from build123d import *

# Parameters (mm, degrees)
SKETCH_1_R          = 10
EXTRUDE_1_DEPTH     = 30
SKETCH_2_R          = 1.85
CUT_EXTRUDE_1_DEPTH = 34.166247904
SKETCH_3_R          = 1.85
SKETCH_3_R_2        = 1.6
EXTRUDE_2_DEPTH     = 15
CUT_EXTRUDE_START   = -15
SKETCH_4_R          = 2.5
SKETCH_4_R_2        = 1.85
CUT_EXTRUDE_2_DEPTH = 15
EXTRUDE_START       = -15
SKETCH_5_R          = 1.85
SKETCH_5_R_2        = 1.6
EXTRUDE_3_DEPTH     = 15
SKETCH_6_R          = 2.5
CUT_EXTRUDE_4_DEPTH = 15
SKETCH_8_W          = 25
SKETCH_8_H          = 25
SKETCH_8_R          = 10
EXTRUDE_4_DEPTH     = 3
FILLET_1_R          = 4
FILLET_6_R          = 12.5
FILLET_7_R          = 12.5
FILLET_8_R          = 12.5
FILLET_9_R          = 12.5
EXTRUDE_START_2     = -25
SKETCH_9_R          = 2.5
EXTRUDE_6_DEPTH     = 25
SKETCH_10_R         = 1.9
CUT_EXTRUDE_5_DEPTH = 10
SKETCH_11_R         = 3
CUT_EXTRUDE_6_DEPTH = 15
EXTRUDE_START_3     = 20
SKETCH_13_R         = 10
SKETCH_13_R_2       = 3
SKETCH_13_R_3       = 1.9
EXTRUDE_7_DEPTH     = 20


# Some blends are built 0.0001 mm under size
with BuildPart() as part:
    # 草图1 → 凸台-拉伸1 (new body)
    with BuildSketch(Plane(origin=(0, 0, 0), x_dir=(1, 0, 0), z_dir=(0, 1, 0))):
        with Locations(Location((0, 0, 0), (0, 0, 270))):
            Circle(SKETCH_1_R)
    extrude(amount=EXTRUDE_1_DEPTH)

    # 草图2 → 切除-拉伸1 (cut, through all)
    with BuildSketch(Plane(origin=(0, 30, 0), x_dir=(1, 0, 0), z_dir=(0, 1, 0))):
        with Locations(Location((0, 6, 0), (0, 0, 270))):
            Circle(SKETCH_2_R)
        with Locations(Location((5.196152423, 3, 0), (0, 0, 270))):
            Circle(SKETCH_2_R)
        with Locations(Location((5.196152423, -3, 0), (0, 0, 270))):
            Circle(SKETCH_2_R)
        with Locations(Location((0, -6, 0), (0, 0, 270))):
            Circle(SKETCH_2_R)
        with Locations(Location((-5.196152423, -3, 0), (0, 0, 270))):
            Circle(SKETCH_2_R)
        with Locations(Location((-5.196152423, 3, 0), (0, 0, 270))):
            Circle(SKETCH_2_R)
    extrude(amount=-CUT_EXTRUDE_1_DEPTH, mode=Mode.SUBTRACT)

    # 草图3 → 凸台-拉伸2 (add)
    # profile 1 of 3: a face of its own
    with BuildSketch(Plane(origin=(0, 30, 0), x_dir=(1, 0, 0), z_dir=(0, 1, 0))):
        with Locations(Location((0, 6, 0), (0, 0, 270))):
            Circle(SKETCH_3_R)
        with Locations(Location((0, 6, 0), (0, 0, 270))):
            Circle(SKETCH_3_R_2, mode=Mode.SUBTRACT)
    # profile 2 of 3: a face of its own
    with BuildSketch(Plane(origin=(0, 30, 0), x_dir=(1, 0, 0), z_dir=(0, 1, 0))):
        with Locations(Location((-5.196152423, -3, 0), (0, 0, 270))):
            Circle(SKETCH_3_R)
        with Locations(Location((-5.196152423, -3, 0), (0, 0, 270))):
            Circle(SKETCH_3_R_2, mode=Mode.SUBTRACT)
    # profile 3 of 3: a face of its own
    with BuildSketch(Plane(origin=(0, 30, 0), x_dir=(1, 0, 0), z_dir=(0, 1, 0))):
        with Locations(Location((5.196152423, -3, 0), (0, 0, 270))):
            Circle(SKETCH_3_R)
        with Locations(Location((5.196152423, -3, 0), (0, 0, 270))):
            Circle(SKETCH_3_R_2, mode=Mode.SUBTRACT)
    extrude(amount=-EXTRUDE_2_DEPTH)

    # 草图4 → 切除-拉伸2 (cut)
    # profile 1 of 3: a face of its own
    with BuildSketch(Plane.XZ.offset(CUT_EXTRUDE_START)):
        with Locations(Location((-5.196152423, 3, 0), (0, 0, 270))):
            Circle(SKETCH_4_R)
        with Locations((-5.196152423, 3)):
            Circle(SKETCH_4_R_2, mode=Mode.SUBTRACT)
    # profile 2 of 3: a face of its own
    with BuildSketch(Plane.XZ.offset(CUT_EXTRUDE_START)):
        with Locations(Location((5.196152423, 3, 0), (0, 0, 270))):
            Circle(SKETCH_4_R)
        with Locations((5.196152423, 3)):
            Circle(SKETCH_4_R_2, mode=Mode.SUBTRACT)
    # profile 3 of 3: a face of its own
    with BuildSketch(Plane.XZ.offset(CUT_EXTRUDE_START)):
        with Locations(Location((0, -6, 0), (0, 0, 270))):
            Circle(SKETCH_4_R)
        with Locations((0, -6)):
            Circle(SKETCH_4_R_2, mode=Mode.SUBTRACT)
    extrude(amount=CUT_EXTRUDE_2_DEPTH, mode=Mode.SUBTRACT)

    # 草图5 → 凸台-拉伸3 (add)
    # profile 1 of 3: a face of its own
    with BuildSketch(Plane.XZ.offset(EXTRUDE_START)):
        with Locations(Location((0, 6, 0), (0, 0, 90))):
            Circle(SKETCH_5_R)
        with Locations(Location((0, 6, 0), (0, 0, 270))):
            Circle(SKETCH_5_R_2, mode=Mode.SUBTRACT)
    # profile 2 of 3: a face of its own
    with BuildSketch(Plane.XZ.offset(EXTRUDE_START)):
        with Locations(Location((-5.196152423, -3, 0), (0, 0, 90))):
            Circle(SKETCH_5_R)
        with Locations(Location((-5.196152423, -3, 0), (0, 0, 270))):
            Circle(SKETCH_5_R_2, mode=Mode.SUBTRACT)
    # profile 3 of 3: a face of its own
    with BuildSketch(Plane.XZ.offset(EXTRUDE_START)):
        with Locations(Location((5.196152423, -3, 0), (0, 0, 90))):
            Circle(SKETCH_5_R)
        with Locations(Location((5.196152423, -3, 0), (0, 0, 270))):
            Circle(SKETCH_5_R_2, mode=Mode.SUBTRACT)
    extrude(amount=EXTRUDE_3_DEPTH)

    # 草图6 → 切除-拉伸4 (cut)
    with BuildSketch(Plane(origin=(0, 30, 0), x_dir=(1, 0, 0), z_dir=(0, 1, 0))):
        with Locations(Location((-5.196152423, 3, 0), (0, 0, 270))):
            Circle(SKETCH_6_R)
        with Locations(Location((5.196152423, 3, 0), (0, 0, 270))):
            Circle(SKETCH_6_R)
        with Locations(Location((0, -6, 0), (0, 0, 270))):
            Circle(SKETCH_6_R)
    extrude(amount=-CUT_EXTRUDE_4_DEPTH, mode=Mode.SUBTRACT)

    # 草图8 → 凸台-拉伸4 (add)
    with BuildSketch(Plane.XZ):
        Rectangle(SKETCH_8_W, SKETCH_8_H)
        with Locations(Location((0, 0, 0), (0, 0, 270))):
            Circle(SKETCH_8_R, mode=Mode.SUBTRACT)
    extrude(amount=-EXTRUDE_4_DEPTH)

    # 圆角1
    # the kernel refuses this fillet: 4 mm, written as the material it adds along each edge
    with BuildSketch(Plane(origin=(0, 3, 0), x_dir=(0, 0, 1), z_dir=(-1, 0, 0))) as fillet_1_piece_1_section:
        with BuildLine():
            CenterArc((10 + FILLET_1_R, FILLET_1_R), FILLET_1_R, 180, 90)
            Line((10 + FILLET_1_R, 0), (10, 0))
            Line((10, 0), (10, FILLET_1_R))
        make_face()
    fillet_1_piece_1 = revolve(axis=Axis((0, 3, 0), (0, 1, 0)), mode=Mode.PRIVATE)
    fillet_1_piece_1 = split(fillet_1_piece_1, bisect_by=Plane(origin=(-12.5, 4.125745955, -11.125745955), z_dir=(1, 0, 0)), keep=Keep.TOP, mode=Mode.PRIVATE)
    fillet_1_piece_1 = split(fillet_1_piece_1, bisect_by=Plane(origin=(0, 4.125745955, 12.5), z_dir=(0, 0, -1)), keep=Keep.TOP, mode=Mode.PRIVATE)
    fillet_1_piece_1 = split(fillet_1_piece_1, bisect_by=Plane(origin=(12.5, 4.125745955, -11.125745955), z_dir=(-1, 0, 0)), keep=Keep.TOP, mode=Mode.PRIVATE)
    fillet_1_piece_1 = split(fillet_1_piece_1, bisect_by=Plane(origin=(0, 4.125745955, -12.5), z_dir=(0, 0, 1)), keep=Keep.TOP, mode=Mode.PRIVATE)
    add(fillet_1_piece_1)

    # 圆角6
    fillet_6_edges = [part.edges().sort_by_distance(p)[0] for p in [
        (12.5, 1.5, 12.5),
    ]]
    fillet(fillet_6_edges, radius=FILLET_6_R)

    # 圆角7
    fillet_7_edges = [part.edges().sort_by_distance(p)[0] for p in [
        (-12.5, 1.5, 12.5),
    ]]
    fillet(fillet_7_edges, radius=FILLET_7_R - 0.0001)  # a hair under: the kernel refuses the full size

    # 圆角8
    fillet_8_edges = [part.edges().sort_by_distance(p)[0] for p in [
        (-12.5, 1.5, -12.5),
    ]]
    fillet(fillet_8_edges, radius=FILLET_8_R)

    # 圆角9
    fillet_9_edges = [part.edges().sort_by_distance(p)[0] for p in [
        (12.5, 1.5, -12.5),
    ]]
    fillet(fillet_9_edges, radius=FILLET_9_R - 0.0001)  # a hair under: the kernel refuses the full size

    # 草图9 → 凸台-拉伸6 (add)
    with BuildSketch(Plane.XZ.offset(EXTRUDE_START_2)):
        with Locations((5.196152423, 3)):
            Circle(SKETCH_9_R)
        with Locations((-5.196152423, 3)):
            Circle(SKETCH_9_R)
        with Locations((0, -6)):
            Circle(SKETCH_9_R)
    extrude(amount=EXTRUDE_6_DEPTH)

    # 草图10 → 切除-拉伸5 (cut)
    with BuildSketch(Plane(origin=(0, 30, 0), x_dir=(1, 0, 0), z_dir=(0, 1, 0))):
        with Locations(Location((0, 6, 0), (0, 0, 270))):
            Circle(SKETCH_10_R)
        with Locations(Location((-5.196152423, -3, 0), (0, 0, 270))):
            Circle(SKETCH_10_R)
        with Locations(Location((5.196152423, -3, 0), (0, 0, 270))):
            Circle(SKETCH_10_R)
    extrude(amount=-CUT_EXTRUDE_5_DEPTH, mode=Mode.SUBTRACT)

    # 草图11 → 切除-拉伸6 (cut)
    with BuildSketch(Plane(origin=(0, 30, 0), x_dir=(1, 0, 0), z_dir=(0, 1, 0))):
        with Locations(Location((-5.196152423, 3, 0), (0, 0, 270))):
            Circle(SKETCH_11_R)
        with Locations(Location((5.196152423, 3, 0), (0, 0, 270))):
            Circle(SKETCH_11_R)
        with Locations(Location((0, -6, 0), (0, 0, 270))):
            Circle(SKETCH_11_R)
    extrude(amount=-CUT_EXTRUDE_6_DEPTH, mode=Mode.SUBTRACT)

    # 草图13 → 凸台-拉伸7 (add)
    with BuildSketch(Plane(origin=(0, 30, 0), x_dir=(1, 0, 0), z_dir=(0, 1, 0)).offset(EXTRUDE_START_3)):
        with Locations(Location((0, 0, 0), (0, 0, 270))):
            Circle(SKETCH_13_R)
        with Locations(Location((-5.196152423, 3, 0), (0, 0, 270))):
            Circle(SKETCH_13_R_2, mode=Mode.SUBTRACT)
        with Locations(Location((0, 6, 0), (0, 0, 270))):
            Circle(SKETCH_13_R_3, mode=Mode.SUBTRACT)
        with Locations(Location((5.196152423, 3, 0), (0, 0, 270))):
            Circle(SKETCH_13_R_2, mode=Mode.SUBTRACT)
        with Locations(Location((0, -6, 0), (0, 0, 270))):
            Circle(SKETCH_13_R_2, mode=Mode.SUBTRACT)
        with Locations(Location((5.196152423, -3, 0), (0, 0, 270))):
            Circle(SKETCH_13_R_3, mode=Mode.SUBTRACT)
        with Locations(Location((-5.196152423, -3, 0), (0, 0, 270))):
            Circle(SKETCH_13_R_3, mode=Mode.SUBTRACT)
    extrude(amount=-EXTRUDE_7_DEPTH)


solid = part.part
The listing builds one solid part. Answer for the finished solid, in the listing's coordinates (mm). A direction names the side the tool comes from. Round coordinates to 2 decimals unless told otherwise and drop trailing zeros. Write each loop counter-clockwise with the first axis right and the second up, starting at its lowest first coordinate (ties: lowest second). Pieces come first, ordered by that corner, then holes. Notation, with made-up numbers: M 67,-40 L 93,-40 A19 cw 93,-22 Z; hole C 65,28 d10. An arc over 180 degrees is marked long. Write each question's results on one line, items separated by ' | '. Start each with the question number.
Item 1: Find section C-C on y = 17. Write down the section's boundary in (x, z).
Item 2: Straight lines are drawn through the part: probe 1 along X at (y, z) = (32, -3); probe 2 along Z at (x, y) = (-5.25, 29); probe 3 along Z at (x, y) = (5, 44.5). For each, find the intervals that lie inside material, in ascending order.
Item 3: Given pin 1 Ø1.9 at (x, z) = (-5.5, 3.5) entering from +Y; pin 2 Ø4 at (x, z) = (5.2, -3) entering from +Y; pin 3 Ø1 at (x, y) = (4, 39) entering from +Z, each flat-ended and moving along its own axis, determine where each tip first touches the part or whether it passes through.
Item 4: Which of the six approach directions +Z, -Z, +X, -X, +Y, -Y give full straight-line access (tool end or side, diameter ignored) to faces 4 (the flat face through (0, 0, 0)), 5 (the flat face through (0, 20, -6))?
Item 5: Find section A-A on y = 40. Write down the section's boundary in (x, z).
Item 6: The mould has two halves that part along X. Classify faces 1 (the flat face through (6.5, 15, -1.7)), 2 (the flat face through (0, 50, 0)), 3 (the cylindrical face through (8.741, 1.669, -8.936)): +X half, -X half, draft (parallel to the pull), parting line (faces both ways), or undercut.
Item 7: Find section B-B on z = -3. Give the number of separate pieces and of enclosed holes in the cut face, and give its area (3 significant figures).
Answer block:
1) outline: C 0,0 d20; hole C -5.2,-3 d6; hole C 0,6 d6; hole C 5.2,-3 d6
2) probe 1: x = -9.54 to -8.2, -2.2 to 2.2, 8.2 to 9.54 | probe 2: z = -8.51 to -6, 0 to 1.1, 4.9 to 8.51 | probe 3: z = -8.66 to -5.99, -0.01 to 1.11, 4.89 to 8.66
3) pin 1: stops at y = 20 | pin 2: stops at y = 15 | pin 3: stops at z = 9.37
4) face 4: +Z, -Z, +X, -X, -Y | face 5: +Y
5) outline: C 0,0 d20; hole C -5.2,-3 d6; hole C -5.2,3 d3.8; hole C 0,6 d6; hole C 0,-6 d3.8; hole C 5.2,-3 d6; hole C 5.2,3 d3.8
6) face 1: undercut | face 2: draft | face 3: +X half
7) separate pieces: 3 | enclosed holes: 0 | area: 460 mm²
